Source: CAD feature listing. Evaluate the final solid. Frame: model axes, mm. A direction names the side the tool comes from. Coordinates: 2 decimals unless noted, no trailing zeros. Order: outer loops, then holes, each group sorted by start corner. A loop starts at its lowest first (then second) coordinate and runs counter-clockwise, first axis right, second up.
Item 1: Reachability of faces 1 (the cylindrical face through (64, 108, 3)), 2 (the flat face through (77, 110, 2)), 3 (the flat face through (-80, 87, 2)) from +Z, -Z, +X, -X, +Y, -Y: full face, straight path, thin tool, end or side. Return the list, or none.
Item 2: Ray query, line 1 (Y direction, x = 0, z = 3.45); line 2 (X direction, y = 80, z = 2.25); line 3 (X direction, y = 29, z = 3.1). Return the intervals inside material, ascending.
Item 3: Section B-B on y = 55. Return the cut outline in (x, z).
Item 4: Section D-D on z = 1.55. State how many separate pieces and enclosed holes the cut face has, then the cut area to 3 significant figures.
Item 5: Section A-A on x = -60.5. Return the cut outline in (y, z), then the cut area to 3 significant figures.
Item 6: Contact query for a flat-ended pin moving along its axis: P1, Ø2.5, axis at x = -82.5, y = -80, coming from the +Z side. Output: stop coordinate, or through.
Item 7: Section C-C on x = 0. Return the cut outline in (y, z).
Item 8: Mould query, pull axis Y, two halves, no side actions, for faces 4 (the flat face through (80, 72, 2)), 5 (the flat face through (-1, -110, 2)), 6 (the cylindrical face through (-88, 109, 3)), 7 (the flat face through (70, 55, 2)). Classes: released by +Y, released by -Y, zero draft, split by the parting line, or undercut.
from build123d import *

# Parameters (mm, degrees)
BOSS_EXTRUDE1_OUTLINE_W   = 5
BOSS_EXTRUDE1_OUTLINE_H   = 5
BOSS_EXTRUDE1_OUTLINE_R   = 1.5
BOSS_EXTRUDE1_OUTLINE_R_2 = 5
BOSS_EXTRUDE1_DEPTH       = 5
FILLET1_R                 = 5


# Read off the part's stored shape, not the designer's step: Boss-Extrude1
with BuildPart() as part:
    # Boss-Extrude1 outline → Boss-Extrude1 (new body)
    with BuildSketch(Plane.XY):
        Polygon((-63, 110), (-90, 110), (-90, -110), (90, -110), (90, 110), (63, 110), (63, 100), (-63, 100), align=None)
        with Locations((-82.5, -102.5)):
            Rectangle(BOSS_EXTRUDE1_OUTLINE_W, BOSS_EXTRUDE1_OUTLINE_H, mode=Mode.SUBTRACT)
        with Locations((-75, -102.5)):
            Circle(BOSS_EXTRUDE1_OUTLINE_R, mode=Mode.SUBTRACT)
        with Locations((-82.5, -87.5)):
            Rectangle(BOSS_EXTRUDE1_OUTLINE_W, BOSS_EXTRUDE1_OUTLINE_H, mode=Mode.SUBTRACT)
        with Locations((-67.5, -102.5)):
            Rectangle(BOSS_EXTRUDE1_OUTLINE_W, BOSS_EXTRUDE1_OUTLINE_H, mode=Mode.SUBTRACT)
        with Locations((-82.5, -80)):
            Circle(BOSS_EXTRUDE1_OUTLINE_R, mode=Mode.SUBTRACT)
        with Locations((-82.5, -72.5)):
            Rectangle(BOSS_EXTRUDE1_OUTLINE_W, BOSS_EXTRUDE1_OUTLINE_H, mode=Mode.SUBTRACT)
        with Locations((0, -85)):
            Circle(BOSS_EXTRUDE1_OUTLINE_R_2, mode=Mode.SUBTRACT)
        with Locations((67.5, -102.5)):
            Rectangle(BOSS_EXTRUDE1_OUTLINE_W, BOSS_EXTRUDE1_OUTLINE_H, mode=Mode.SUBTRACT)
        with Locations((75, -102.5)):
            Circle(BOSS_EXTRUDE1_OUTLINE_R, mode=Mode.SUBTRACT)
        with Locations((82.5, -102.5)):
            Rectangle(BOSS_EXTRUDE1_OUTLINE_W, BOSS_EXTRUDE1_OUTLINE_H, mode=Mode.SUBTRACT)
        with Locations((82.5, -87.5)):
            Rectangle(BOSS_EXTRUDE1_OUTLINE_W, BOSS_EXTRUDE1_OUTLINE_H, mode=Mode.SUBTRACT)
        with Locations((82.5, -80)):
            Circle(BOSS_EXTRUDE1_OUTLINE_R, mode=Mode.SUBTRACT)
        with Locations((82.5, -72.5)):
            Rectangle(BOSS_EXTRUDE1_OUTLINE_W, BOSS_EXTRUDE1_OUTLINE_H, mode=Mode.SUBTRACT)
        with Locations((-82.5, 72.5)):
            Rectangle(BOSS_EXTRUDE1_OUTLINE_W, BOSS_EXTRUDE1_OUTLINE_H, mode=Mode.SUBTRACT)
        with Locations((-82.5, 80)):
            Circle(BOSS_EXTRUDE1_OUTLINE_R, mode=Mode.SUBTRACT)
        with Locations((-82.5, 87.5)):
            Rectangle(BOSS_EXTRUDE1_OUTLINE_W, BOSS_EXTRUDE1_OUTLINE_H, mode=Mode.SUBTRACT)
        with Locations((-82.5, 102.5)):
            Rectangle(BOSS_EXTRUDE1_OUTLINE_W, BOSS_EXTRUDE1_OUTLINE_H, mode=Mode.SUBTRACT)
        with Locations((-75, 102.5)):
            Circle(BOSS_EXTRUDE1_OUTLINE_R, mode=Mode.SUBTRACT)
        with Locations((-67.5, 102.5)):
            Rectangle(BOSS_EXTRUDE1_OUTLINE_W, BOSS_EXTRUDE1_OUTLINE_H, mode=Mode.SUBTRACT)
        with BuildLine():
            Line((70, 20), (24.979991994, 20))
            ThreePointArc((24.979991994, 20), (0, -32), (-24.979991994, 20))
            Line((-24.979991994, 20), (-70, 20))
            Line((-70, 20), (-70, 90))
            Line((-70, 90), (70, 90))
            Line((70, 90), (70, 20))
        make_face(mode=Mode.SUBTRACT)
        with Locations((82.5, 72.5)):
            Rectangle(BOSS_EXTRUDE1_OUTLINE_W, BOSS_EXTRUDE1_OUTLINE_H, mode=Mode.SUBTRACT)
        with Locations((82.5, 80)):
            Circle(BOSS_EXTRUDE1_OUTLINE_R, mode=Mode.SUBTRACT)
        with Locations((82.5, 87.5)):
            Rectangle(BOSS_EXTRUDE1_OUTLINE_W, BOSS_EXTRUDE1_OUTLINE_H, mode=Mode.SUBTRACT)
        with Locations((67.5, 102.5)):
            Rectangle(BOSS_EXTRUDE1_OUTLINE_W, BOSS_EXTRUDE1_OUTLINE_H, mode=Mode.SUBTRACT)
        with Locations((75, 102.5)):
            Circle(BOSS_EXTRUDE1_OUTLINE_R, mode=Mode.SUBTRACT)
        with Locations((82.5, 102.5)):
            Rectangle(BOSS_EXTRUDE1_OUTLINE_W, BOSS_EXTRUDE1_OUTLINE_H, mode=Mode.SUBTRACT)
    extrude(amount=BOSS_EXTRUDE1_DEPTH)

    # Fillet1
    fillet1_edges = [part.edges().sort_by_distance(p)[0] for p in [
        (-63, 110, 2.5),
        (63, 110, 2.5),
        (90, 110, 2.5),
        (90, -110, 2.5),
        (-90, -110, 2.5),
        (-90, 110, 2.5),
        (-24.979991994, 20, 2.5),
        (24.979991994, 20, 2.5),
        (70, 20, 2.5),
        (70, 90, 2.5),
        (-70, 90, 2.5),
        (-70, 20, 2.5),
    ]]
    fillet(fillet1_edges, radius=FILLET1_R)


solid = part.part
Answer list:
1. face 1: +Z, -Z, +Y
1. face 2: +Z, -Z, +X, -X, +Y
1. face 3: +Z, -Z
2. line 1: y = -110 to -90, -80 to -32, 90 to 100
2. line 2: x = -90 to -84, -81 to -70, 70 to 81, 84 to 90
2. line 3: x = -90 to -70, 70 to 90
3. outline: (-90, 0) - (-70, 0) - (-70, 5) - (-90, 5) - close; (70, 0) - (90, 0) - (90, 5) - (70, 5) - close
4. separate pieces: 1
4. enclosed holes: 26
4. area: 25,200 mm2
5. outline: (-110, 0) - (20, 0) - (20, 5) - (-110, 5) - close; (90, 0) - (100, 0) - (100, 5) - (90, 5) - close
5. area: 700 mm2
6. P1: passes through
7. outline: (-110, 0) - (-90, 0) - (-90, 5) - (-110, 5) - close; (-80, 0) - (-32, 0) - (-32, 5) - (-80, 5) - close; (90, 0) - (100, 0) - (100, 5) - (90, 5) - close
8. face 4: undercut
8. face 5: released by -Y
8. face 6: released by +Y
8. face 7: undercut
